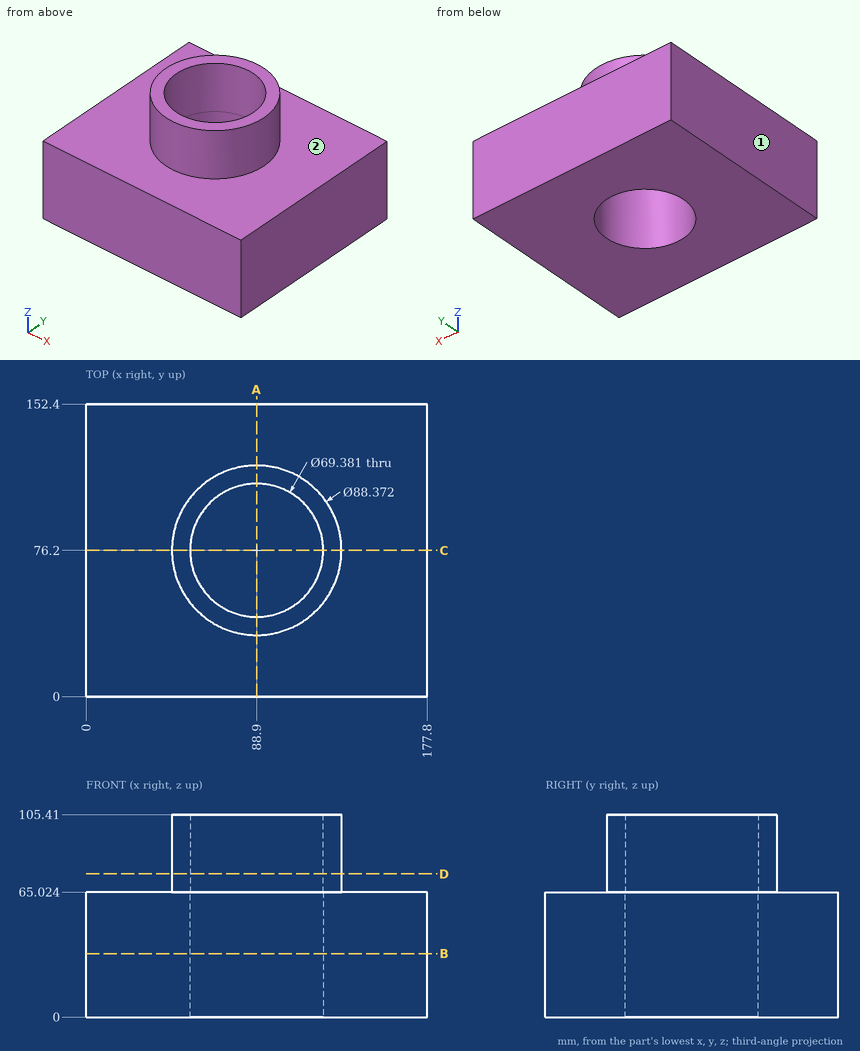
Part print with two shaded views. Sizes in mm from the minimum x, y, z corner. A direction names the side the tool comes from. Round coordinates to 2 decimals unless told otherwise and drop trailing zeros. Loops run counter-clockwise (first coordinate to the right, second up) from the corner with the lowest first, then second, coordinate; pieces in that order, holes last.
Item 1: Drill centre lines: line 1 along Y through (x, z) = (88.9, 46.5); line 2 along Y through (x, z) = (88, 83); line 3 along Z through (x, y) = (139, 93.5). Where is each one in solid material? Low to high.
Item 2: Which spindle directions (+Z, -Z, +X, -X, +Y, -Y) get a long thin tool onto all of the face, cutting with end or side? Do the marked faces 1 and 2. Say none if no direction does.
Item 3: Saw through at B-B (z = 33). List the corners of the cut face in (x, y), then the cut area to 3 significant figures.
Item 4: Saw through at D-D (z = 74.5). List the corners of the cut face in (x, y), then the cut area to 3 significant figures.
Item 5: Pin check, flat tips, straight feed: P1, Ø12, axis at x = 111.5, z = 88.5, coming from the +Y side; P2, Ø8, axis at x = 21.5, y = 29.5, coming from the +Z side; P3, Ø3, axis at y = 62.5, z = 91, coming from the -X side. Stop position of each tip, or through.
Item 6: Saw through at C-C (y = 76.2). List the corners of the cut face in (x, z).
Item 7: Saw through at A-A (x = 88.9). List the corners of the cut face in (y, z), then the cut area to 3 significant figures.
Worked answers:
1. line 1: y = 0 to 41.51, 110.89 to 152.4
1. line 2: y = 32.02 to 41.52, 110.88 to 120.38
1. line 3: z = 0 to 65.02
2. face 1: +Z, -Z, -X, +Y, -Y
2. face 2: +Z
3. outline: (0, 0) - (177.8, 0) - (177.8, 152.4) - (0, 152.4) - close; hole circle Ø69.38 at (88.9, 76.2)
3. area: 23,300 mm2
4. outline: circle Ø88.37 at (88.9, 76.2); hole circle Ø69.38 at (88.9, 76.2)
4. area: 2,350 mm2
5. P1: stops at y = 117.15
5. P2: stops at z = 65.02
5. P3: stops at x = 46.43
6. outline: (0, 0) - (54.21, 0) - (54.21, 105.41) - (44.71, 105.41) - (44.71, 65.02) - (0, 65.02) - close; (123.59, 0) - (177.8, 0) - (177.8, 65.02) - (133.09, 65.02) - (133.09, 105.41) - (123.59, 105.41) - close
7. outline: (0, 0) - (41.51, 0) - (41.51, 105.41) - (32.01, 105.41) - (32.01, 65.02) - (0, 65.02) - close; (110.89, 0) - (152.4, 0) - (152.4, 65.02) - (120.39, 65.02) - (120.39, 105.41) - (110.89, 105.41) - close
7. area: 6,170 mm2
